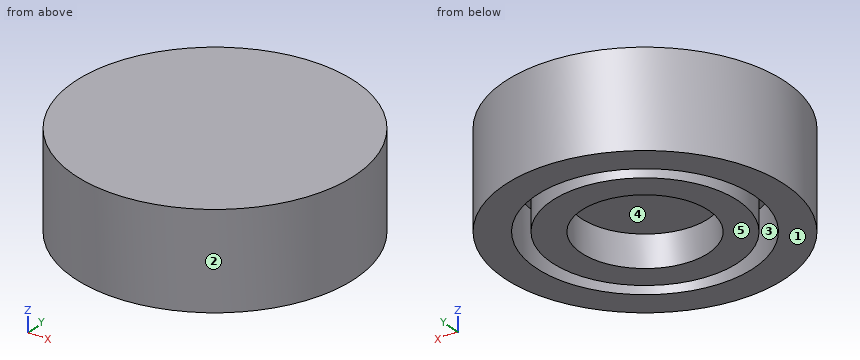
```python
from build123d import *

# Parameters (mm, degrees)
SKETCH1_R           = 22
BOSS_EXTRUDE1_DEPTH = 15
SKETCH2_R           = 10
CUT_EXTRUDE1_DEPTH  = 5
SKETCH3_R           = 17.075773731
SKETCH3_R_2         = 14.593062164
CUT_EXTRUDE2_DEPTH  = 8


with BuildPart() as part:
    # Sketch1 → Boss-Extrude1 (new body)
    with BuildSketch(Plane.XY):
        Circle(SKETCH1_R)
    extrude(amount=BOSS_EXTRUDE1_DEPTH)

    # Sketch2 → Cut-Extrude1 (cut)
    with BuildSketch(Plane(origin=(0, 0, 0), x_dir=(-1, 0, 0), z_dir=(0, 0, -1))):
        Circle(SKETCH2_R)
    extrude(amount=-CUT_EXTRUDE1_DEPTH, mode=Mode.SUBTRACT)

    # Sketch3 → Cut-Extrude2 (cut)
    with BuildSketch(Plane(origin=(0, 0, 0), x_dir=(-1, 0, 0), z_dir=(0, 0, -1))):
        Circle(SKETCH3_R)
        Circle(SKETCH3_R_2, mode=Mode.SUBTRACT)
    extrude(amount=-CUT_EXTRUDE2_DEPTH, mode=Mode.SUBTRACT)


solid = part.part
```
Here's how the part is built. I have some questions about the finished solid (model axes, mm). Face numbers are marked on the shaded views. A direction names the side the tool comes from. Give positions to 0.01 mm unless a question says otherwise; leave off trailing zeros. Write each loop counter-clockwise with the first axis right and the second up, starting at its lowest first coordinate (ties: lowest second). Pieces come first, ordered by that corner, then holes. Notation, with made-up numbers: (-39, 9.5) -> (1, 9.5) arc R11 cw to (1, 20.5) -> close; hole circle Ø10 at (89.25, 61). An arc over 180 degrees is marked (long way). Use one line per item in the form item = value.
1) On a 3-axis mill with a long thin cutter (end or side, diameter ignored), from which of +Z, -Z, +X, -X, +Y, -Y can I reach the whole of each face in a straight line? I mean the marked faces 4 and 5. Say none if no direction works.
Verdict:
face_4 = -Z
face_5 = -Z, +X, -X, +Y, -Y
2) If I drill on L1, parallel to Y at x = 0, z = 1.2; L2, parallel to Y at x = 0, z = 6; L3, parallel to Y at x = 11.5, z = 2.25 (3 decimals), over which ranges is the centre line in solid material (lowest first)? Write a range as [from, to].
Verdict:
L1 = [-22, -17.08], [-14.59, -10], [10, 14.59], [17.08, 22]
L2 = [-22, -17.08], [-14.59, 14.59], [17.08, 22]
L3 = [-18.755, -12.623], [-8.984, 8.984], [12.623, 18.755]
3) We'd pull the mould along Y, two halves only. Please class the marked faces 1, 2 and 3: +Y half, -Y half, draft (parallel to the pull), parting line (faces both ways), or undercut.
Verdict:
face_1 = draft
face_2 = parting line
face_3 = undercut
4) Suppose I cut it at A-A (z = 1.5). Please give me the cut outline in (x, y), and give its area (3 significant figures).
Verdict:
outline = circle Ø44 at (0, 0); circle Ø29.19 at (0, 0); hole circle Ø34.15 at (0, 0); hole circle Ø20 at (0, 0)
area = 959 mm2
5) Suppose I cut it at D-D (y = 16). Please give me the cut outline in (x, z), and give its area (3 significant figures).
Verdict:
outline = (-15.1, 0) -> (-5.97, 0) -> (-5.97, 8) -> (5.97, 8) -> (5.97, 0) -> (15.1, 0) -> (15.1, 15) -> (-15.1, 15) -> close
area = 358 mm2
6) I'm going to push flat-ended pins straight in: pin 1 (6 mm diameter, centred on x = -5.5, z = 4.5, fed in from +Y); pin 2 (16 mm diameter, centred on x = 0, y = 0, fed in from -Z); pin 3 (4 mm diameter, centred on x = -12, z = 6.5, fed in from -Y). Where does each tip first touch, or does it pass through?
Verdict:
pin_1 = 21.86
pin_2 = 5
pin_3 = -19.6
7) Suppose I cut it at B-B (x = 0). Please give me the cut outline in (y, z), and give its area (3 significant figures).
Verdict:
outline = (-22, 0) -> (-17.08, 0) -> (-17.08, 8) -> (-14.59, 8) -> (-14.59, 0) -> (-10, 0) -> (-10, 5) -> (10, 5) -> (10, 0) -> (14.59, 0) -> (14.59, 8) -> (17.08, 8) -> (17.08, 0) -> (22, 0) -> (22, 15) -> (-22, 15) -> close
area = 520 mm2
